Part model, mm, in its own coordinate system. A direction names the side the tool comes from. Round coordinates to 2 decimals unless told otherwise and drop trailing zeros. Order: outer loops, then holes, each group sorted by start corner. A loop starts at its lowest first (then second) coordinate and runs counter-clockwise, first axis right, second up. Notation, with made-up numbers: M 25.5,28 L 51.5,28 A20 ccw 51.5,65 Z; hole C 9,10.25 d9. An arc over 180 degrees is marked long. One line per question, with ' | ' between items.
from build123d import *

# Parameters (mm, degrees)
F0_R     = 25
F1_DEPTH = 10
F2_W     = 18.193654716
F2_H     = 28.7717729807
F3_DEPTH = 50
F4_R     = 1
F5_R     = 2


with BuildPart() as f1:
    # F0 (on Front) → F1 (new body, symmetric)
    with BuildSketch(Plane.XZ):
        Circle(F0_R)
    extrude(amount=F1_DEPTH, both=True)

    # F2 (on face) → F3 (join)
    with BuildSketch(Plane.XZ.offset(10)):
        Rectangle(F2_W, F2_H)
    extrude(amount=F3_DEPTH)

    # F4
    f4_edges = [f1.edges().sort_by_distance(p)[0] for p in [
        (0, -10, 14.385886),
        (9.096827, -10, 0),
        (-9.096827, -10, 0),
        (0, -10, -14.385886),
        (-9.096827, -35, -14.385886),
        (-9.096827, -35, 14.385886),
        (9.096827, -35, 14.385886),
        (9.096827, -35, -14.385886),
        (9.096827, -60, 0),
        (-9.096827, -60, 0),
        (0, -60, 14.385886),
        (0, -60, -14.385886),
    ]]
    fillet(f4_edges, radius=F4_R)

    # F5
    f5_edges = [f1.edges().sort_by_distance(p)[0] for p in [
        (0, -10, 15.385886),
        (9.511041, -10, 14.8001),
        (-9.511041, -10, 14.8001),
        (10.096827, -10, 0),
        (-10.096827, -10, 0),
        (9.511041, -10, -14.8001),
        (-9.511041, -10, -14.8001),
        (0, -10, -15.385886),
        (-25, -10, 0),
    ]]
    fillet(f5_edges, radius=F5_R)


solid = f1.part
1) Saw through at C-C (x = 0). List the corners of the cut face in (y, z).
The answers:
outline: M -60,-13.39 A1 ccw -59,-14.39 L -11,-14.39 A1 cw -10,-15.39 L -10,-23 A2 ccw -8,-25 L 10,-25 L 10,25 L -8,25 A2 ccw -10,23 L -10,15.39 A1 cw -11,14.39 L -59,14.39 A1 ccw -60,13.39 Z
2) Probe line 1 (Y direction, x = 18.5, z = 1.5); line 2 (Z direction, x = 4.5, y = -47); line 3 (X direction, y = -6, z = 0.5) (3 decimals). List the from-to ranges inside material, lowest first. Write a range as [from, to].
The answers:
line 1: y = [-10, 10] | line 2: z = [-14.39, 14.39] | line 3: x = [-24.995, 24.995]
3) Saw through at B-B (z = 0). List the corners of the cut face in (x, y).
The answers:
outline: M -25,-8 A2 ccw -23,-10 L -10.1,-10 A1 cw -9.1,-11 L -9.1,-59 A1 ccw -8.1,-60 L 8.1,-60 A1 ccw 9.1,-59 L 9.1,-11 A1 cw 10.1,-10 L 23,-10 A2 ccw 25,-8 L 25,10 L -25,10 Z
4) Drop flat-ended pins along their axis: pin 1 (21.5 mm diameter, centred on y = -23.5, z = 2, fed in from +X); pin 2 (4 mm diameter, centred on y = -20, z = 12, fed in from -X); pin 3 (10 mm diameter, centred on x = -10, z = -4, fed in from -Y); pin 4 (3 mm diameter, centred on x = -11.5, y = -9, fed in from +Z). Give the stop position or say it passes through.
The answers:
pin 1: stops at x = 9.1 | pin 2: stops at x = -9.1 | pin 3: stops at y = -60 | pin 4: stops at z = 22.81
5) Which spindle directions (+Z, -Z, +X, -X, +Y, -Y) get a long thin tool onto all of the face, cutting with end or side? Do faces 1 (the face through (0, -35, 14.386)), 2 (the face through (-9.097, -35, 0)), 3 (the face through (9.097, -35, 0)), 4 (the face through (0, -35, -14.386)). Say none if no direction does.
The answers:
face 1: +Z, +X, -X, -Y | face 2: +Z, -Z, -X, -Y | face 3: +Z, -Z, +X, -Y | face 4: -Z, +X, -X, -Y
6) Saw through at A-A (y = -41). List the corners of the cut face in (x, z).
The answers:
outline: M -9.1,-13.39 A1 ccw -8.1,-14.39 L 8.1,-14.39 A1 ccw 9.1,-13.39 L 9.1,13.39 A1 ccw 8.1,14.39 L -8.1,14.39 A1 ccw -9.1,13.39 Z
